```python
from build123d import *

# Parameters (mm, degrees)
ESTRUSIONE_ESTRUSIONE1_DEPTH = 38
TAGLIO_ESTRUSIONE1_DEPTH     = 32
TAGLIO_ESTRUSIONE3_DEPTH     = 48.370877129
TAGLIO_ESTRUSIONE4_DEPTH     = 53.671149598
TAGLIO_ESTRUSIONE5_DEPTH     = 53.671149598


with BuildPart() as part:
    # Schizzo2 → Estrusione-Estrusione1 (new body)
    with BuildSketch(Plane(origin=(0, 0, 0), x_dir=(0, 0, -1), z_dir=(1, 0, 0))):
        Polygon((-20, -20), (20, -20), (20, 20), align=None)
    extrude(amount=ESTRUSIONE_ESTRUSIONE1_DEPTH)

    # Schizzo3 → Taglio-Estrusione1 (cut)
    with BuildSketch(Plane(origin=(35, 0, 0), x_dir=(0, 0, -1), z_dir=(1, 0, 0))):
        Polygon((-20, -14.5), (14.5, 20), (14.5, -14.5), align=None)
    extrude(amount=-TAGLIO_ESTRUSIONE1_DEPTH, mode=Mode.SUBTRACT)

    # Schizzo5 → Taglio-Estrusione3 (cut, through all)
    with BuildSketch(Plane(origin=(0, 0, 0), x_dir=(0, 0, -1), z_dir=(1, 0, 0))):
        Polygon((16, 16), (20, 16), (20, 20), align=None)
        Polygon((-20, -20), (-16, -16), (-16, -20), align=None)
    extrude(amount=TAGLIO_ESTRUSIONE3_DEPTH, mode=Mode.SUBTRACT)

    # Schizzo6 → Taglio-Estrusione4 (cut, through all)
    with BuildSketch(Plane.XY.offset(-14.5)):
        Polygon((25.6, 9.5), (12.4, 9.5), (12.4, 0.8), (14.65, 0.8), (14.65, -10.5), (23.35, -10.5), (23.35, 0.8), (25.6, 0.8), align=None)
    extrude(amount=-TAGLIO_ESTRUSIONE4_DEPTH, mode=Mode.SUBTRACT)

    # Schizzo8 → Taglio-Estrusione5 (cut, through all)
    with BuildSketch(Plane(origin=(0, -14.5, 0), x_dir=(1, 0, 0), z_dir=(0, 1, 0))):
        Polygon((25.6, -9.5), (12.4, -9.5), (12.4, -0.8), (14.65, -0.8), (14.65, 10.5), (23.35, 10.5), (23.35, -0.8), (25.6, -0.8), align=None)
    extrude(amount=-TAGLIO_ESTRUSIONE5_DEPTH, mode=Mode.SUBTRACT)


solid = part.part
```
Check sheet for the modelled part. Datum: model origin and axes. Units: mm. A direction names the side the tool comes from. Round coordinates to 2 decimals unless told otherwise and drop trailing zeros. Loops run counter-clockwise (first coordinate to the right, second up) from the corner with the lowest first, then second, coordinate; pieces in that order, holes last. Notation, with made-up numbers: (37.5, 29.25) -> (61.5, 29.25) arc R32 ccw to (61.5, 58.25) -> close; hole circle Ø4 at (21, -5). An arc over 180 degrees is marked (long way). Answer in a Markdown table with one row per item.
Q1. Sectioned sample at D-D on x = 30. Enter the section's corners in (y, z).
Data:
| item | result |
|---|---|
| outline | (-20, -20) -> (16, -20) -> (16, -16) -> (14.5, -14.5) -> (-14.5, -14.5) -> (-14.5, 14.5) -> (-16, 16) -> (-20, 16) -> close |
Q2. Sectioned sample at A-A on z = 3.5. Enter the section's corners in (x, y), then the cut area to 3 significant figures.
Data:
| item | result |
|---|---|
| outline | (0, -20) -> (12.4, -20) -> (12.4, -14.5) -> (3, -14.5) -> (3, -3.5) -> (0, -3.5) -> close; (25.6, -20) -> (38, -20) -> (38, -3.5) -> (35, -3.5) -> (35, -14.5) -> (25.6, -14.5) -> close |
| area | 202 mm^2 |
Q3. Release check for a two-part mould opening along X. For faces 4 (the face through (19, 16, -18)), 5 (the face through (24, -17, 0.8)), 6 (the face through (0, -6, -6)) record: released by +X, released by -X, zero draft, split by the parting line, or undercut.
Data:
| item | result |
|---|---|
| face 4 | zero draft |
| face 5 | undercut |
| face 6 | released by -X |
Q4. Sectioned sample at C-C on y = -1. Enter the section's corners in (x, z).
Data:
| item | result |
|---|---|
| outline | (0, -20) -> (14.65, -20) -> (14.65, -14.5) -> (3, -14.5) -> (3, 1) -> (0, 1) -> close; (23.35, -20) -> (38, -20) -> (38, 1) -> (35, 1) -> (35, -14.5) -> (23.35, -14.5) -> close |
Q5. Sectioned sample at B-B on x = 20. Enter the section's corners in (y, z), then the cut area to 4 significant figures.
Data:
| item | result |
|---|---|
| outline | (-20, -20) -> (-10.5, -20) -> (-10.5, -14.5) -> (-14.5, -14.5) -> (-14.5, -10.5) -> (-20, -10.5) -> close; (-20, 9.5) -> (-14.5, 9.5) -> (-14.5, 14.5) -> (-16, 16) -> (-20, 16) -> close; (9.5, -20) -> (16, -20) -> (16, -16) -> (14.5, -14.5) -> (9.5, -14.5) -> close |
| area | 143.5 mm^2 |
Q6. Thickness scan on L1, parallel to X at y = 6, z = -13.5; L2, parallel to X at y = -1, z = -18; L3, parallel to Y at x = 34, z = 12.5. Record the ranges inside material, lowest first.
Data:
| item | result |
|---|---|
| L1 | x = 0 to 3, 35 to 38 |
| L2 | x = 0 to 14.65, 23.35 to 38 |
| L3 | y = -20 to -14.5 |
Q7. Set-up check for faces 1 (the face through (23.35, -17, -5)), 2 (the face through (3, -6, -7)), 3 (the face through (19, -10.5, -17)): record each of +Z, -Z, +X, -X, +Y, -Y from which the full face is reachable in a straight line by a thin tool's end or side.
Data:
| item | result |
|---|---|
| face 1 | +Y, -Y |
| face 2 | +Z, +Y |
| face 3 | +Z, -Z |
